Read the model definition and answer for the solid it produces. Units are mm, in the model's axes. Coordinates: 2 decimals unless noted, no trailing zeros. Write each loop counter-clockwise with the first axis right and the second up, starting at its lowest first coordinate (ties: lowest second). Pieces come first, ordered by that corner, then holes. Notation, with made-up numbers: (89, 30.25) -> (146, 30.25) arc R20 cw to (146, 44.25) -> close; hole circle Ø2 at (-10, 20). An arc over 180 degrees is marked (long way). Answer in a Markdown table with one row per item. Add a question column.
Item 1: Section B-B on y = -10 is taken. Write down the section's boundary in (x, z), then the cut area to 3 significant figures.
Item 2: Section A-A on x = 1 is taken. Write down the section's boundary in (y, z).
Item 3: Section C-C on z = 1.2 is taken. Write down the section's boundary in (x, y).
Item 4: Straight lines are drawn through the part: line 1 (Y direction, x = -17, z = 1.4); line 2 (X direction, y = -28.5, z = 1.9); line 3 (X direction, y = -7.5, z = 1.15). For each, find the intervals that lie inside material, in ascending order. Write a range as from..to.
Item 5: Section D-D on x = -32.5 is taken. Write down the section's boundary in (y, z), then the cut area to 3 significant figures.
Item 6: For a pull along Y with two mould halves and no side action, classify faces 1 (the face through (-14.308, -47.175, 0.986)), 2 (the face through (34.305, -13, 1)), 3 (the face through (-6, 28.854, 1)), 4 (the face through (1.56, -6.76, 1.01)) as +Y half, -Y half, draft (parallel to the pull), parting line (faces both ways), or undercut.
```python
from build123d import *

# Parameters (mm, degrees)
ESBO_O1_W                  = 74
ESBO_O1_H                  = 77
RESSALTO_EXTRUS_O1_DEPTH   = 2
ESBO_O2_R                  = 13.5
CORTE_EXTRUS_O2_DEPTH      = 2
CORTE_EXTRUS_O4_DEPTH      = 1
CORTE_EXTRUS_O4_DEPTH_BACK = 3
FILETE1_R                  = 5
FILETE3_R                  = 10
FILETE4_R                  = 10


with BuildPart() as part:
    # Esboço1 → Ressalto-extrusão1 (new body)
    with BuildSketch(Plane.XY):
        with Locations((-2.694889042, -9.645522388)):
            Rectangle(ESBO_O1_W, ESBO_O1_H)
    extrude(amount=RESSALTO_EXTRUS_O1_DEPTH)

    # Esboço2 → Corte-extrusão2 (cut)
    with BuildSketch(Plane.XY.offset(2)):
        with Locations((-5.694889042, -18.145522388)):
            Circle(ESBO_O2_R)
    extrude(amount=-CORTE_EXTRUS_O2_DEPTH, mode=Mode.SUBTRACT)

    # Esboço3 → Corte-extrusão4 (cut, two sides)
    with BuildSketch(Plane.XY.offset(2)) as corte_extrus_o4_sk:
        Polygon((-162.954500024, 129.766010791), (-39.694889042, -18.145522388), (-14.694889042, -48.145522388), (108.564721941, -196.057055567), (-187.258344417, -442.576277532), (-458.777566382, -116.753211174), align=None)
    extrude(amount=CORTE_EXTRUS_O4_DEPTH, mode=Mode.SUBTRACT)
    extrude(corte_extrus_o4_sk.sketch, amount=-CORTE_EXTRUS_O4_DEPTH_BACK, mode=Mode.SUBTRACT)

    # Filete1
    filete1_edges = [part.edges().sort_by_distance(p)[0] for p in [
        (34.305110958, 28.854477612, 1),
    ]]
    fillet(filete1_edges, radius=FILETE1_R)

    # Filete3
    filete3_edges = [part.edges().sort_by_distance(p)[0] for p in [
        (-39.694889042, -18.145522388, 1),
    ]]
    fillet(filete3_edges, radius=FILETE3_R)

    # Filete4
    filete4_edges = [part.edges().sort_by_distance(p)[0] for p in [
        (-14.694889042, -48.145522388, 1),
    ]]
    fillet(filete4_edges, radius=FILETE4_R)


solid = part.part
```
Results below:
| question | item | result |
|---|---|---|
| 1 | outline | (-39.69, 0) -> (-16.46, 0) -> (-16.46, 2) -> (-39.69, 2) -> close; (5.07, 0) -> (34.31, 0) -> (34.31, 2) -> (5.07, 2) -> close |
| 1 | area | 105 mm2 |
| 2 | outline | (-48.15, 0) -> (-29.87, 0) -> (-29.87, 2) -> (-48.15, 2) -> close; (-6.42, 0) -> (28.85, 0) -> (28.85, 2) -> (-6.42, 2) -> close |
| 3 | outline | (-39.69, -14.53) arc R10 ccw to (-37.38, -20.93) -> (-17.69, -44.55) arc R10 ccw to (-10.01, -48.15) -> (34.31, -48.15) -> (34.31, 23.85) arc R5 ccw to (29.31, 28.85) -> (-39.69, 28.85) -> close; hole circle Ø27 at (-5.69, -18.15) |
| 4 | line 1 | y = -45.3..-25.52, -10.77..28.85 |
| 4 | line 2 | x = -31.07..-14.36, 2.97..34.31 |
| 4 | line 3 | x = -39.69..-14, 2.61..34.31 |
| 5 | outline | (-26.78, 0) -> (28.85, 0) -> (28.85, 2) -> (-26.78, 2) -> close |
| 5 | area | 111 mm2 |
| 6 | face 1 | -Y half |
| 6 | face 2 | draft |
| 6 | face 3 | +Y half |
| 6 | face 4 | undercut |
